Part model, mm, in its own coordinate system. A direction names the side the tool comes from. Round coordinates to 2 decimals unless told otherwise and drop trailing zeros. Loops run counter-clockwise (first coordinate to the right, second up) from the corner with the lowest first, then second, coordinate; pieces in that order, holes last. Notation, with made-up numbers: (25, 57) - (58, 57) arc R13 ccw to (58, 67) - close; hole circle Ø3 at (-9, 10). An arc over 180 degrees is marked (long way). Put each result on its own line as item: value.
from build123d import *

# Parameters (mm, degrees)
SKETCH1_R                               = 40
SKETCH1_R_2                             = 20
BOSS_EXTRUDE1_DEPTH                     = 8.5
SKETCH2_R                               = 1
CUT_EXTRUDE2_DEPTH                      = 58.203583804
SKETCH2_6_R                             = 3
SKETCH2_6_R_2                           = 1
BOSS_EXTRUDE3_DEPTH                     = 8.5
CIRPATTERN1_COUNT                       = 4
CUT_EXTRUDE4_DEPTH                      = 62.402361518
CIRPATTERN3_COUNT                       = 4
SKETCH7_R                               = 21
CUT_EXTRUDE5_DEPTH                      = 7
SKETCH8_R                               = 1
OUTER_RETAINER_M2_TAPPED_ENVELOPE_DEPTH = 4.3


with BuildPart() as part:
    # Sketch1 → Boss-Extrude1 (new body)
    with BuildSketch(Plane(origin=(0, 0, 0), x_dir=(1, 0, 0), z_dir=(0, 1, 0))):
        with Locations(Location((0, 0, 0), (0, 0, 270))):
            Circle(SKETCH1_R)
        with Locations(Location((0, 0, 0), (0, 0, 270))):
            Circle(SKETCH1_R_2, mode=Mode.SUBTRACT)
    extrude(amount=BOSS_EXTRUDE1_DEPTH)

    # Sketch2 → Cut-Extrude2 (cut, through all)
    with BuildSketch(Plane(origin=(0, 8.5, 0), x_dir=(1, 0, 0), z_dir=(0, 1, 0))):
        with Locations((40, 0)):
            Circle(SKETCH2_R)
    cut_extrude2 = extrude(amount=-CUT_EXTRUDE2_DEPTH, mode=Mode.SUBTRACT)

    # Sketch2_6 → Boss-Extrude3 (add)
    with BuildSketch(Plane(origin=(0, 8.5, 0), x_dir=(1, 0, 0), z_dir=(0, 1, 0))):
        with Locations((40, 0)):
            Circle(SKETCH2_6_R)
        with Locations(Location((40, 0, 0), (0, 0, 270))):
            Circle(SKETCH2_6_R_2, mode=Mode.SUBTRACT)
    boss_extrude3 = extrude(amount=-BOSS_EXTRUDE3_DEPTH)

    # CirPattern1: Cut-Extrude2, Boss-Extrude3 ×4 about axis
    cirpattern1_axis = Axis((0, 0, 0), (0, 1, 0))
    add([cut_extrude2.rotate(cirpattern1_axis, i * 360 / CIRPATTERN1_COUNT) for i in range(1, CIRPATTERN1_COUNT)], mode=Mode.SUBTRACT)
    add([boss_extrude3.rotate(cirpattern1_axis, i * 360 / CIRPATTERN1_COUNT) for i in range(1, CIRPATTERN1_COUNT)])

    # Sketch4 → Cut-Extrude4 (cut, through all)
    with BuildSketch(Plane(origin=(0, 8.5, 0), x_dir=(1, 0, 0), z_dir=(0, 1, 0))):
        with BuildLine():
            Line((-27.170578067, -25.049257724), (-17.377149148, -15.255828804))
            ThreePointArc((-17.377149148, -15.255828804), (-15.255828804, -15.255828804), (-15.255828804, -17.377149148))
            Line((-15.255828804, -17.377149148), (-25.049257724, -27.170578067))
            ThreePointArc((-25.049257724, -27.170578067), (-27.170578067, -27.170578067), (-27.170578067, -25.049257724))
        make_face()
    cut_extrude4 = extrude(amount=-CUT_EXTRUDE4_DEPTH, mode=Mode.SUBTRACT)

    # CirPattern3: Cut-Extrude4 ×4 about axis
    cirpattern3_axis = Axis((0, 0, 0), (0, 1, 0))
    for i in range(1, CIRPATTERN3_COUNT):
        add(cut_extrude4.rotate(cirpattern3_axis, i * 360 / CIRPATTERN3_COUNT), mode=Mode.SUBTRACT)

    # Sketch7 → Cut-Extrude5 (cut)
    with BuildSketch(Plane(origin=(0, 8.5, 0), x_dir=(1, 0, 0), z_dir=(0, 1, 0))):
        with Locations(Location((0, 0, 0), (0, 0, 270))):
            Circle(SKETCH7_R)
    extrude(amount=-CUT_EXTRUDE5_DEPTH, mode=Mode.SUBTRACT)

    # Sketch8 → Outer_Retainer_M2_Tapped_Envelope (cut)
    with BuildSketch(Plane(origin=(0, 8.5, 0), x_dir=(1, 0, 0), z_dir=(0, 1, 0))):
        with Locations(Location((0.720053396, -22.48847534, 0), (0, 0, 270))):
            Circle(SKETCH8_R)
        with Locations(Location((19.115564239, 11.867822203, 0), (0, 0, 270))):
            Circle(SKETCH8_R)
        with Locations(Location((-19.835617634, 10.620653137, 0), (0, 0, 270))):
            Circle(SKETCH8_R)
    extrude(amount=-OUTER_RETAINER_M2_TAPPED_ENVELOPE_DEPTH, mode=Mode.SUBTRACT)


solid = part.part
1. Band-saw the part on D-D (x = -32). List the corners of the cut face in (y, z).
A:
outline: (0, -24) - (8.5, -24) - (8.5, 24) - (0, 24) - close
2. Band-saw the part on C-C (z = -22.5). List the corners of the cut face in (x, y), plus the area to 3 significant figures.
A:
outline: (-33.07, 0) - (-24.62, 0) - (-24.62, 8.5) - (-33.07, 8.5) - close; (-20.38, 0) - (20.38, 0) - (20.38, 8.5) - (-20.38, 8.5) - close; (24.62, 0) - (33.07, 0) - (33.07, 8.5) - (24.62, 8.5) - close
area: 490 mm²
3. Pin check, flat tips, straight feed: P1, Ø2, axis at y = 4, z = 33.5, coming from the +X side; P2, Ø4, axis at x = -6, y = 1, coming from the -Z side; P3, Ø5, axis at y = 3, z = -8, coming from the -X side. Stop position of each tip, or through.
A:
P1: stops at x = 23.32
P2: stops at z = -39.8
P3: stops at x = -39.62
4. Band-saw the part on B-B (y = 6.75). Give the number of separate pieces and of enclosed holes in the cut face, plus the area to 3 significant figures.
A:
separate pieces: 1
enclosed holes: 12
area: 3,480 mm²
5. Probe line 1 along X through (y, z) = (3.25, 17.5); line 2 along Z through (x, y) = (40, 4.75); line 3 along X through (y, z) = (2.25, 25). List the from-to ranges inside material, lowest first. Write a range as [from, to].
A:
line 1: x = [-35.97, -19.62], [-15.38, -11.61], [11.61, 15.38], [19.62, 35.97]
line 2: z = [-3, -1], [1, 3]
line 3: x = [-31.22, -27.12], [-22.88, 22.88], [27.12, 31.22]
6. Two-plate mould, pull along X, no slides. Class faces 4 (the cylindrical face through (0, 4, 43)), 5 (the cylindrical face through (28.002, 4.19, 28.564)), 6 (the cylindrical face through (27.15, 4.31, -27.19)), 7 (the cylindrical face through (-15.28, 4.31, 15.23)): pulls with the +X half, pulls with the -X half, needs draft (parallel to the pull), parting line crosses it, or undercut.
A:
face 4: parting line crosses it
face 5: pulls with the +X half
face 6: undercut
face 7: undercut
7. Band-saw the part on A-A (z = 0). List the corners of the cut face in (x, y).
A:
outline: (-43, 0) - (-41, 0) - (-41, 8.5) - (-43, 8.5) - close; (-39, 0) - (-20, 0) - (-20, 1.5) - (-21, 1.5) - (-21, 8.5) - (-39, 8.5) - close; (20, 0) - (39, 0) - (39, 8.5) - (21, 8.5) - (21, 1.5) - (20, 1.5) - close; (41, 0) - (43, 0) - (43, 8.5) - (41, 8.5) - close
8. Tool access for faces 1 (the flat face through (-20.22, 4.31, -22.34)), 2 (the cylindrical face through (0.76, 6.38, 21.49)), 3 (the cylindrical face through (-28.002, 4.19, -28.564)): list every direction of +Z, -Z, +X, -X, +Y, -Y with a clear straight run to the whole face (end or side of a thin tool).
A:
face 1: +Y, -Y
face 2: +Y
face 3: -Z, -X, +Y, -Y
